from build123d import *

# Parameters (mm, degrees)
SKETCH1_W           = 280
SKETCH1_H           = 35
SKETCH1_R           = 2.08
SKETCH1_R_2         = 6
SKETCH1_R_3         = 4
BOSS_EXTRUDE1_DEPTH = 6


with BuildPart() as part:
    # Sketch1 → Boss-Extrude1 (new body)
    with BuildSketch(Plane(origin=(0, 0, 0), x_dir=(1, 0, 0), z_dir=(0, 1, 0))):
        Rectangle(SKETCH1_W, SKETCH1_H)
        with Locations((40, 5)):
            Circle(SKETCH1_R, mode=Mode.SUBTRACT)
        with Locations((-40, 5)):
            Circle(SKETCH1_R, mode=Mode.SUBTRACT)
        Circle(SKETCH1_R_2, mode=Mode.SUBTRACT)
        with Locations((10, 10)):
            Circle(SKETCH1_R, mode=Mode.SUBTRACT)
        with Locations((-10, 10)):
            Circle(SKETCH1_R, mode=Mode.SUBTRACT)
        with Locations((-10, -10)):
            Circle(SKETCH1_R, mode=Mode.SUBTRACT)
        with Locations((10, -10)):
            Circle(SKETCH1_R, mode=Mode.SUBTRACT)
        with Locations((120, 10)):
            Circle(SKETCH1_R_3, mode=Mode.SUBTRACT)
        with Locations((-120, 10)):
            Circle(SKETCH1_R_3, mode=Mode.SUBTRACT)
        with Locations((120, -10)):
            Circle(SKETCH1_R_3, mode=Mode.SUBTRACT)
        with Locations((-120, -10)):
            Circle(SKETCH1_R_3, mode=Mode.SUBTRACT)
    extrude(amount=BOSS_EXTRUDE1_DEPTH)


solid = part.part
The model under review builds one solid part; all positions refer to its coordinate system, in mm. Round coordinates to 2 decimals unless told otherwise and drop trailing zeros. Write each loop counter-clockwise with the first axis right and the second up, starting at its lowest first coordinate (ties: lowest second). Pieces come first, ordered by that corner, then holes. Notation, with made-up numbers: M -10,16.25 L -1,16.25 A15 cw -1,21.25 Z; hole C 51.5,25.25 d6. An arc over 180 degrees is marked long. Answer as CSV lines item,"result". Start each with the question number.
Q1. Consider section B-B, the plane z = 0. Give the boundary of the cut face in (x, y), then the cut area to 3 significant figures.
Q2. The part is to be moulded in two halves that separate along Z. For faces 1 (the face through (-140, 3, 0)), 2 (the face through (-116.305, 2.958, 11.532)), 3 (the face through (-2, 3, 17.5)), 4 (the face through (-116.185, 2.958, -11.201)), say which applies: +Z half, -Z half, draft (parallel to the pull), parting line (faces both ways), or undercut.
Q3. Consider section C-C, the plane y = 1.9. State how many separate pieces and enclosed holes the cut face has, then the cut area to 3 significant figures.
Q4. Consider section A-A, the plane x = 120. Give the boundary of the cut face in (y, z), then the cut area to 3 significant figures.
Q5. Wall thickness on line 1 along Z through (x, y) = (10, 2); line 2 along X through (y, z) = (3.3, -10); line 3 along Z through (x, y) = (-120, 4.45): over which ranges is each line inside the solid? List them lowest first.
Result set:
1,outline,"M -140,0 L -6,0 L -6,6 L -140,6 Z; M 6,0 L 140,0 L 140,6 L 6,6 Z"
1,area,"1,610 mm²"
2,face 1,"draft"
2,face 2,"undercut"
2,face 3,"+Z half"
2,face 4,"undercut"
3,separate pieces,"1"
3,enclosed holes,"11"
3,area,"9,400 mm²"
4,outline,"M 0,-17.5 L 6,-17.5 L 6,-14 L 0,-14 Z; M 0,-6 L 6,-6 L 6,6 L 0,6 Z; M 0,14 L 6,14 L 6,17.5 L 0,17.5 Z"
4,area,"114 mm²"
5,line 1,"z = -17.5 to -12.08, -7.92 to 7.92, 12.08 to 17.5"
5,line 2,"x = -140 to -124, -116 to -12.08, -7.92 to 7.92, 12.08 to 116, 124 to 140"
5,line 3,"z = -17.5 to -14, -6 to 6, 14 to 17.5"
